Geometry check sheet. Reference: drawing and pictorial views, mm from the part's lowest x, y, z. A direction names the side the tool comes from. Round coordinates to 2 decimals unless told otherwise and drop trailing zeros. Loops run counter-clockwise (first coordinate to the right, second up) from the corner with the lowest first, then second, coordinate; pieces in that order, holes last. Notation, with made-up numbers: M 18.5,-26.5 L 62.5,-26.5 A14 ccw 62.5,-12.5 Z; hole C 31.25,-23.5 d10. An arc over 180 degrees is marked long. One line per question, with ' | ' between items. Start each with the question number.
(1) Go/stop test with flat-tipped pins: P1, Ø6, axis at x = 6.5, z = 42, coming from the +Y side; P2, Ø2, axis at x = 32, z = 27.5, coming from the +Y side. Record where each tip stops, or that it passes through.
(2) Section check C-C (z = 22). Record the boundary of the cut face in (x, y), and give its area (3 significant figures).
(3) Draft check along X on the marked faces 1, 2 and 3. Enter one of: +X half, -X half, draft (parallel to the pull), parting line (faces both ways), or undercut.
(4) Tool access check on the marked faces 4 and 5. Record the directions out of +Z, -Z, +X, -X, +Y, -Y that give a thin tool (end or side, any length) a straight path to the whole face; none if there is none.
(5) Section check A-A (y = 41.5). Record the boundary of the cut face in (x, z).
(6) Section check B-B (x = 28). Record the boundary of the cut face in (y, z).
(7) Thickness scan on probe 1 along X at (y, z) = (4.2, 38); probe 2 along X at (y, z) = (62, 19); probe 3 along Z at (x, y) = (1.5, 57). Record the ranges inside material, lowest first. Write a range as [from, to].
(8) Section check D-D (y = 57). Record the boundary of the cut face in (x, z).
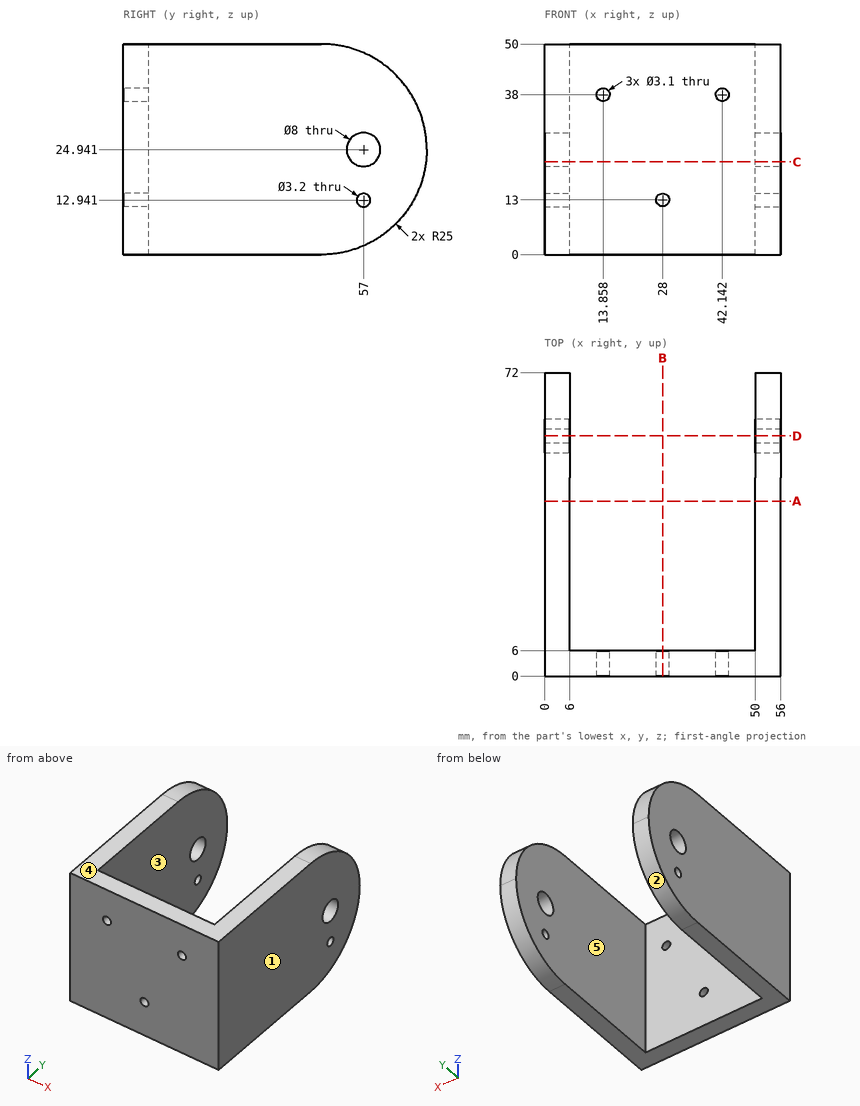
The answers:
1) P1: y = 67.68 | P2: y = 6
2) outline: M 0,0 L 56,0 L 56,54.29 L 50,54.29 L 50,6 L 6,6 L 6,54.29 L 0,54.29 Z; M 0,59.71 L 6,59.71 L 6,71.82 L 0,71.82 Z; M 50,59.71 L 56,59.71 L 56,71.82 L 50,71.82 Z | area: 1,060 mm²
3) face 1: +X half | face 2: draft | face 3: undercut
4) face 4: +Z, +X, -X, +Y, -Y | face 5: +Z, -Z, +Y
5) outline: M 0,0 L 6,0 L 6,50 L 0,50 Z; M 50,0 L 56,0 L 56,50 L 50,50 Z
6) outline: M 0,0 L 6,0 L 6,11.45 L 0,11.45 Z; M 0,14.55 L 6,14.55 L 6,50 L 0,50 Z
7) probe 1: [0, 12.31], [15.41, 40.59], [43.69, 56] | probe 2: [0, 6], [50, 56] | probe 3: [2.09, 11.34], [14.54, 20.94], [28.94, 47.91]
8) outline: M 0,2.09 L 6,2.09 L 6,11.34 L 0,11.34 Z; M 0,14.54 L 6,14.54 L 6,20.94 L 0,20.94 Z; M 0,28.94 L 6,28.94 L 6,47.91 L 0,47.91 Z; M 50,2.09 L 56,2.09 L 56,11.34 L 50,11.34 Z; M 50,14.54 L 56,14.54 L 56,20.94 L 50,20.94 Z; M 50,28.94 L 56,28.94 L 56,47.91 L 50,47.91 Z
